Check sheet for the modelled part. Datum: model origin and axes. Units: mm. Face numbers are marked on the shaded views. A direction names the side the tool comes from. Give positions to 0.01 mm unless a question says otherwise; leave off trailing zeros. Order: outer loops, then holes, each group sorted by start corner. A loop starts at its lowest first (then second) coordinate and runs counter-clockwise, first axis right, second up.
```python
from build123d import *

# Parameters (mm, degrees)
SKETCH1_W           = 52
SKETCH1_H           = 40
BOSS_EXTRUDE1_DEPTH = 2
SKETCH2_R           = 0.95
CUT_EXTRUDE1_DEPTH  = 33.86335345
BOSS_EXTRUDE2_START = 4
SKETCH3_R           = 2.5
SKETCH3_R_2         = 0.95
BOSS_EXTRUDE2_DEPTH = 4
SKETCH4_W           = 5
SKETCH4_H           = 26
BOSS_EXTRUDE3_DEPTH = 4
SKETCH5_W           = 37
SKETCH5_H           = 25
CUT_EXTRUDE2_DEPTH  = 34.045423284
FILLET1_R           = 2
FILLET2_R           = 6


with BuildPart() as part:
    # Sketch1 → Boss-Extrude1 (new body)
    with BuildSketch(Plane(origin=(0, 0, 0), x_dir=(1, 0, 0), z_dir=(0, 1, 0))):
        Rectangle(SKETCH1_W, SKETCH1_H)
    extrude(amount=BOSS_EXTRUDE1_DEPTH)

    # Sketch2 → Cut-Extrude1 (cut, through all)
    with BuildSketch(Plane(origin=(0, 2, 0), x_dir=(1, 0, 0), z_dir=(0, 1, 0))):
        with Locations(Location((8, 15, 0), (0, 0, 270))):
            Circle(SKETCH2_R)
        with Locations(Location((-8, 15, 0), (0, 0, 270))):
            Circle(SKETCH2_R)
        with Locations(Location((-21.5, 5.32, 0), (0, 0, 270))):
            Circle(SKETCH2_R)
        with Locations(Location((-21.5, -15, 0), (0, 0, 270))):
            Circle(SKETCH2_R)
    extrude(amount=-CUT_EXTRUDE1_DEPTH, mode=Mode.SUBTRACT)

    # Sketch3 → Boss-Extrude2 (add)
    # profile 1 of 4: a face of its own
    with BuildSketch(Plane(origin=(0, 2, 0), x_dir=(1, 0, 0), z_dir=(0, 1, 0)).offset(BOSS_EXTRUDE2_START)):
        with Locations(Location((-21.5, 5.32, 0), (0, 0, 90))):
            Circle(SKETCH3_R)
        with Locations(Location((-21.5, 5.32, 0), (0, 0, 270))):
            Circle(SKETCH3_R_2, mode=Mode.SUBTRACT)
    # profile 2 of 4: a face of its own
    with BuildSketch(Plane(origin=(0, 2, 0), x_dir=(1, 0, 0), z_dir=(0, 1, 0)).offset(BOSS_EXTRUDE2_START)):
        with Locations(Location((-21.5, -15, 0), (0, 0, 90))):
            Circle(SKETCH3_R)
        with Locations(Location((-21.5, -15, 0), (0, 0, 270))):
            Circle(SKETCH3_R_2, mode=Mode.SUBTRACT)
    # profile 3 of 4: a face of its own
    with BuildSketch(Plane(origin=(0, 2, 0), x_dir=(1, 0, 0), z_dir=(0, 1, 0)).offset(BOSS_EXTRUDE2_START)):
        with Locations(Location((8, 15, 0), (0, 0, 90))):
            Circle(SKETCH3_R)
        with Locations(Location((8, 15, 0), (0, 0, 270))):
            Circle(SKETCH3_R_2, mode=Mode.SUBTRACT)
    # profile 4 of 4: a face of its own
    with BuildSketch(Plane(origin=(0, 2, 0), x_dir=(1, 0, 0), z_dir=(0, 1, 0)).offset(BOSS_EXTRUDE2_START)):
        with Locations(Location((-8, 15, 0), (0, 0, 90))):
            Circle(SKETCH3_R)
        with Locations(Location((-8, 15, 0), (0, 0, 270))):
            Circle(SKETCH3_R_2, mode=Mode.SUBTRACT)
    extrude(amount=-BOSS_EXTRUDE2_DEPTH)

    # Sketch4 → Boss-Extrude3 (add)
    with BuildSketch(Plane(origin=(0, 2, 0), x_dir=(1, 0, 0), z_dir=(0, 1, 0))):
        with Locations((23.5, -7)):
            Rectangle(SKETCH4_W, SKETCH4_H)
    extrude(amount=BOSS_EXTRUDE3_DEPTH)

    # Sketch5 → Cut-Extrude2 (cut, through all)
    with BuildSketch(Plane(origin=(0, 2, 0), x_dir=(1, 0, 0), z_dir=(0, 1, 0))):
        with Locations((2.5, -2.5)):
            Rectangle(SKETCH5_W, SKETCH5_H)
    extrude(amount=-CUT_EXTRUDE2_DEPTH, mode=Mode.SUBTRACT)

    # Fillet1
    fillet1_edges = [part.edges().sort_by_distance(p)[0] for p in [
        (26, 4, -6),
        (21, 4, -6),
        (21, 4, 20),
        (26, 3, 20),
    ]]
    fillet(fillet1_edges, radius=FILLET1_R)

    # Fillet2
    fillet2_edges = [part.edges().sort_by_distance(p)[0] for p in [
        (-16, 1, 15),
        (-16, 1, -10),
        (21, 1, -10),
        (21, 1, 15),
        (-26, 1, 20),
        (-26, 1, -20),
        (26, 1, -20),
    ]]
    fillet(fillet2_edges, radius=FILLET2_R)


solid = part.part
```
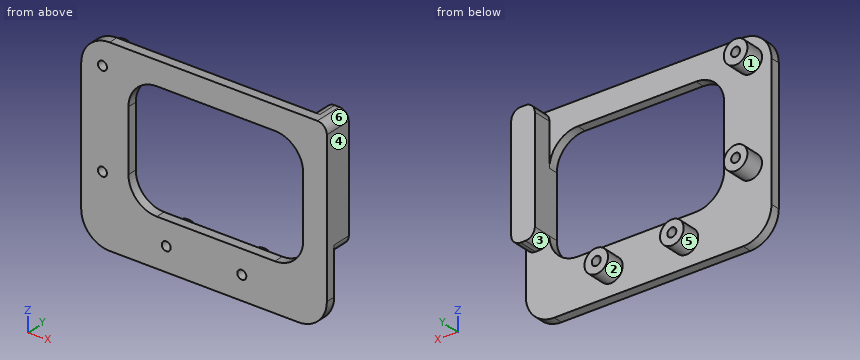
(1) Go/stop test with a flat-tipped pin: P1, Ø1.8, axis at y = 3.5, z = 3.5, coming from the -X side. Record where the tip stops, or that it passes through.
(2) Sectioned sample at B-B (x = 2). Enter the section's corners in (y, z), plus the area to 3 significant figures.
(3) Sectioned sample at C-C (z = -1.5). Enter the section's corners in (x, y), plus the area to 3 significant figures.
(4) Sectioned sample at A-A (y = 4.5). Count the separate pieces of the cut face and the enclosed holes in it, plus the area to 3 significant figures.
(5) Release check for a two-part mould opening along Z. For the marked faces 1, 2, 3 and 4 record: released by +Z, released by -Z, zero draft, split by the parting line, or undercut.
(6) Thickness scan on L1, parallel to X at y = 3.25, z = -15; L2, parallel to X at y = 3.35, z = -5.32; L3, parallel to Z at x = -9, y = 1.6. Record the ranges inside material, lowest first.
(7) Tool access check on the marked faces 5 and 6. Record the directions out of +Z, -Z, +X, -X, +Y, -Y that give a thin tool (end or side, any length) a straight path to the whole face; none if there is none.
(8) Sectioned sample at D-D (x = -8). Enter the section's corners in (y, z), plus the area to 3 significant figures.
Values follow:
1. P1: stops at x = 21
2. outline: (0, -20) - (2, -20) - (2, -10) - (0, -10) - close; (0, 15) - (2, 15) - (2, 20) - (0, 20) - close
2. area: 30.0 mm2
3. outline: (-26, 0) - (-16, 0) - (-16, 2) - (-26, 2) - close; (21, 0) - (26, 0) - (26, 6) - (21, 6) - close
3. area: 50.0 mm2
4. separate pieces: 5
4. enclosed holes: 4
4. area: 194 mm2
5. face 1: undercut
5. face 2: split by the parting line
5. face 3: released by -Z
5. face 4: zero draft
6. L1: x = -10.5 to -8.95, -7.05 to -5.5, 5.5 to 7.05, 8.95 to 10.5
6. L2: x = -24 to -22.45, -20.55 to -19, 21.5 to 25.5
6. L3: z = -20 to -10, 15 to 20
7. face 5: +Y
7. face 6: +Z, +X, +Y, -Y
8. outline: (0, -20) - (2, -20) - (2, -17.5) - (6, -17.5) - (6, -15.95) - (0, -15.95) - close; (0, -14.05) - (6, -14.05) - (6, -12.5) - (2, -12.5) - (2, -10) - (0, -10) - close; (0, 15) - (2, 15) - (2, 20) - (0, 20) - close
8. area: 38.6 mm2
